from build123d import *

# Parameters (mm, degrees)
SKETCH1_R           = 5
SKETCH1_R_2         = 1.8
BOSS_EXTRUDE1_DEPTH = 10
SKETCH2_R           = 12.525
CUT_EXTRUDE1_DEPTH  = 1.425
CHAMFER1_SIZE       = 0.5
CUT_EXTRUDE2_DEPTH  = 2.5
CHAMFER2_SIZE       = 0.5
SKETCH4_R           = 1.8
CUT_EXTRUDE3_DEPTH  = 10
CHAMFER3_SIZE       = 0.5
CHAMFER3_SIZE_2     = 0.923879533
CHAMFER3_SIZE_3     = 0.552958444


with BuildPart() as part:
    # Sketch1 → Boss-Extrude1 (new body)
    with BuildSketch(Plane.XY):
        with BuildLine():
            Line((-40.746699048, 8.183561953), (-33.214821075, -10))
            Line((-33.214821075, -10), (-9.797958971, -10))
            ThreePointArc((-9.797958971, -10), (0, -14), (9.797958971, -10))
            Line((9.797958971, -10), (19.5, -10))
            Line((19.5, -10), (19.5, -3.981225471))
            ThreePointArc((19.5, -3.981225471), (20, 4.0125), (20.5, -3.981225471))
            Line((20.5, -3.981225471), (20.5, -10))
            Line((20.5, -10), (33.214821075, -10))
            Line((33.214821075, -10), (40.746699048, 8.183561953))
            ThreePointArc((40.746699048, 8.183561953), (0, 18.25), (-40.746699048, 8.183561953))
        make_face()
        Circle(SKETCH1_R, mode=Mode.SUBTRACT)
        with Locations((-32.052211881, 8.130884627)):
            Circle(SKETCH1_R_2, mode=Mode.SUBTRACT)
        with Locations(Location((32.052211881, 8.130884627, 0), (0, 0, 180))):
            Circle(SKETCH1_R_2, mode=Mode.SUBTRACT)
        Polygon((-25.988511975, 6.5901118), (-35.250404289, 2.75371039), (-31.414002879, -6.508181923), (-22.152110566, -2.671780514), align=None, mode=Mode.SUBTRACT)
    extrude(amount=BOSS_EXTRUDE1_DEPTH)

    # Sketch2 → Cut-Extrude1 (cut)
    with BuildSketch(Plane.XY.offset(10)):
        Circle(SKETCH2_R)
    extrude(amount=-CUT_EXTRUDE1_DEPTH, mode=Mode.SUBTRACT)

    # Chamfer1
    chamfer1_edges = [part.edges().sort_by_distance(p)[0] for p in [
        (20, 4.0125, 0),
        (-24.070311271, 1.959165643, 0),
        (-30.619458132, 4.671911095, 0),
        (-33.332203584, -1.877235766, 0),
        (-26.783056723, -4.589981218, 0),
    ]]
    chamfer(chamfer1_edges, length=CHAMFER1_SIZE)

    # Sketch3 → Cut-Extrude2 (cut)
    with BuildSketch(Plane.XY.offset(3.75)):
        Polygon((-37.076762037, 12.944469155), (-33.567560961, 4.472508325), (-28.393835579, 6.615535546), (-31.903036655, 15.087496376), align=None)
        Polygon((37.076762037, 12.944469155), (33.567560961, 4.472508325), (28.393835579, 6.615535546), (31.903036655, 15.087496376), align=None)
    extrude(amount=CUT_EXTRUDE2_DEPTH, mode=Mode.SUBTRACT)

    # Chamfer2
    chamfer2_edges = [part.edges().sort_by_distance(p)[0] for p in [
        (14.648979486, -10, 0),
        (0, -14, 0),
        (-21.506390023, -10, 0),
        (-36.980760062, -0.908219024, 0),
        (0, 18.25, 0),
        (36.980760062, -0.908219024, 0),
        (26.857410538, -10, 0),
    ]]
    chamfer(chamfer2_edges, length=CHAMFER2_SIZE)

    # Sketch4 → Cut-Extrude3 (cut)
    with BuildSketch(Plane(origin=(-29.114518455, -12.059628406, 0), x_dir=(0, 0, -1), z_dir=(0.9238795325112882, 0.38268343236508634, 0))):
        with Locations(Location((-5.25, 11.021342374, 0), (0, 0, 90))):
            Circle(SKETCH4_R)
    extrude(amount=-CUT_EXTRUDE3_DEPTH, mode=Mode.SUBTRACT)

    # Chamfer3
    # the kernel refuses this chamfer: 0.923879533, 0.552958444, 0.5 mm, written as the material it takes off along each edge
    with BuildSketch(Plane(origin=(40.746699048, 8.183561953, -0.920037939), x_dir=(-0.38268343236508906, -0.923879532511287, 0), z_dir=(0, 0, 1))) as chamfer3_piece_1:
        with BuildLine():
            Line((CHAMFER3_SIZE, 0), (-0.048717445, -0.548717445))
            ThreePointArc((-0.048717445, -0.548717445), (-0.025540103, -0.282767493), (0, 0))
            Line((0, 0), (CHAMFER3_SIZE, 0))
        make_face()
    extrude(amount=12.340075878, mode=Mode.SUBTRACT)
    with BuildSketch(Plane(origin=(33.214821075, -10, -1.895315111), x_dir=(-1, 0, 0), z_dir=(0, 0, 1))) as chamfer3_piece_2:
        Polygon((CHAMFER3_SIZE, 0), (-CHAMFER3_SIZE_2 * 0.382683432163, -CHAMFER3_SIZE_2 * 0.923879532023), (0, 0), align=None)
    extrude(amount=14.290630221, mode=Mode.SUBTRACT)
    with BuildSketch(Plane(origin=(-33.214821075, -10, -1.895315111), x_dir=(1, 0, 0), z_dir=(0, 0, 1))) as chamfer3_piece_3:
        Polygon((CHAMFER3_SIZE_2, 0), (-CHAMFER3_SIZE * 0.382683432365, CHAMFER3_SIZE * 0.923879532511), (0, 0), align=None)
    extrude(amount=14.290630221, mode=Mode.SUBTRACT)
    with BuildSketch(Plane(origin=(-40.746699048, 8.183561953, -0.925350902), x_dir=(0.38268343236508684, -0.9238795325112881, 0), z_dir=(0, 0, 1))) as chamfer3_piece_4:
        with BuildLine():
            Line((CHAMFER3_SIZE_3, 0), (-0.04424113, 0.496614821))
            ThreePointArc((-0.04424113, 0.496614821), (-0.0231658, 0.256042208), (0, 0))
            Line((0, 0), (CHAMFER3_SIZE_3, 0))
        make_face()
    extrude(amount=12.350701805, mode=Mode.SUBTRACT)


solid = part.part
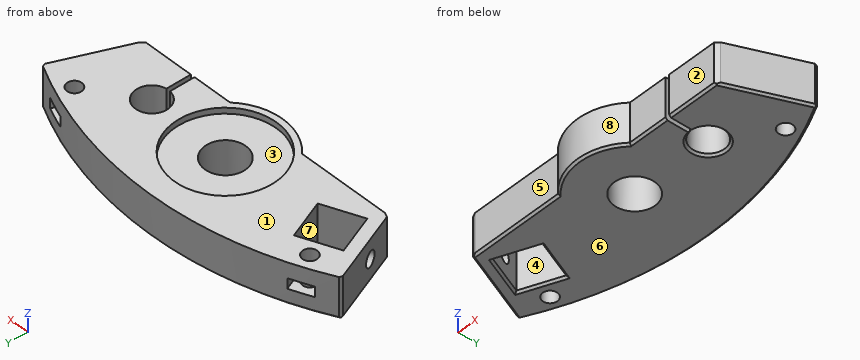
Read the model definition and answer for the solid it produces. Units are mm, in the model's axes. Face numbers are marked on the shaded views. A direction names the side the tool comes from. Round coordinates to 2 decimals unless told otherwise and drop trailing zeros. Write each loop counter-clockwise with the first axis right and the second up, starting at its lowest first coordinate (ties: lowest second). Pieces come first, ordered by that corner, then holes. Notation, with made-up numbers: (-17.5, 0.5) - (24.5, 0.5) arc R29 cw to (24.5, 38.5) - close; hole circle Ø6 at (50.25, 65). An arc over 180 degrees is marked (long way). One line per question, with ' | ' between items. Start each with the question number.
1. Section A-A (x = 0) is taken. Determine the outline of the cut face in (y, z) (3 decimals).
2. For the marked faces 1, 2, 3, 4 and 5, determine the directions among +Z, -Z, +X, -X, +Y, -Y from which every point of the face is accessible in a straight line to the end or side of a thin tool.
3. For a pull along X with two mould halves and no side action, classify the marked faces 6, 7 and 8 as +X half, -X half, draft (parallel to the pull), parting line (faces both ways), or undercut.
4. Find the intervals of material crossed by probe 1 along Y at (x, z) = (-30.5, 8.5); probe 2 along X at (y, z) = (0, 5.75); probe 3 along X at (y, z) = (-5.5, 8.5), in increasing order. Write a range as [from, to].
5. Each of these flat-tipped pins is pushed along its axis until it touches: pin 1 (4 mm diameter, centred on x = 32, y = 7.5, fed in from +Z); pin 2 (3 mm diameter, centred on x = -32.05, y = 8.13, fed in from -Z); pin 3 (6 mm diameter, centred on x = -3, y = -0.5, fed in from +Z) (3 decimals); pin 4 (3 mm diameter, centred on y = -7, z = 7, fed in from -X). Where does it stop, or does it pass through?
Filled in:
1) outline: (-14, 0.5) - (-13.5, 0) - (-5, 0) - (-5, 8.575) - (-12.525, 8.575) - (-12.525, 10) - (-14, 10) - close; (5, 0) - (17.75, 0) - (18.25, 0.5) - (18.25, 10) - (12.525, 10) - (12.525, 8.575) - (5, 8.575) - close
2) face 1: +Z, +X, -X, +Y, -Y | face 2: +Z, -Z, +X, -Y | face 3: +Z | face 4: +Z, -Z | face 5: +Z, -Z, -X, -Y
3) face 6: draft | face 7: undercut | face 8: parting line
4) probe 1: [-10, -6.13], [4.72, 7.22], [9.04, 12.76] | probe 2: [-37.36, -34.11], [-23.26, -5], [5, 15.99], [24.01, 37.36] | probe 3: [-35.08, -31.83], [-28.98, 19.5], [20.5, 35.08]
5) pin 1: z = 10 | pin 2: through | pin 3: z = 8.575 | pin 4: x = -35.08
